Can you work these out from the model? Positions are in its coordinate system, mm. A direction names the side the tool comes from. Coordinates: 2 decimals unless noted, no trailing zeros. Order: outer loops, then holes, each group sorted by start corner. A loop starts at its lowest first (then second) coordinate and runs counter-clockwise, first axis right, second up. Notation, with made-up numbers: (50.25, 35.5) -> (87.25, 35.5) arc R12 ccw to (87.25, 47.5) -> close; hole circle Ø3 at (38, 14). An arc over 180 degrees is marked (long way). Answer in a Markdown table with one row per item. Add a question column.
1. Will these pins go through, and if not, where does the flat tip stop? pin 1 (2 mm diameter, centred on x = -3.5, y = 0.5, fed in from -Z); pin 2 (1.5 mm diameter, centred on x = 5.5, z = -7, fed in from -Y).
2. On a 3-axis mill with a long thin cutter (end or side, diameter ignored), from which of +Z, -Z, +X, -X, +Y, -Y can I reach the whole of each face in a straight line? I mean faces 4 (the face through (-6.987, -2.2, -7.466)), 5 (the face through (6.465, -6.39, -6.42)). Say none if no direction works.
3. If I drill on line 1 along X through (y, z) = (0, -3.5); line 2 along Z through (x, y) = (7.25, 2.25), over which ranges is the centre line in solid material (lowest first)? Write a range as [from, to].
4. Imagine slicing it at C-C on z = -6. Write out the boundary of the cut face in (x, y), plus the area to 3 significant figures.
5. We'd pull the mould along X, two halves only. Please class faces 1 (the face through (0, -9.146, -3)), 2 (the face through (0, 5, -4)), 3 (the face through (6.505, -6.43, -3.197)): pulls with the +X half, pulls with the -X half, needs draft (parallel to the pull), parting line crosses it, or undercut.
Autodesk Inventor part; units mm, degrees
ref_plane "YZ Plane" through (0, 0, 0) normal (1, 0, 0) x (0, 1, 0)
ref_plane "XZ Plane" through (0, 0, 0) normal (0, 1, 0) x (-1, 0, 0)
ref_plane "XY Plane" through (0, 0, 0) normal (0, 0, 1) x (1, 0, 0)
sketch "Sketch1" plane through (0, 0, 0) normal (0, 0, 1) x (1, 0, 0)
  line L0 (-12.8051, 0) -> (12.8051, 0)
  line L1 (9.1465, -3.7886) -> (3.7886, -9.1465)
  line L2 (3.7886, -9.1465) -> (-3.7886, -9.1465)
  line L3 (-3.7886, -9.1465) -> (-9.1465, -3.7886)
  line L4 (-9.1465, -3.7886) -> (-9.1465, 3.7886)
  line L5 (-9.1465, 3.7886) -> (-3.7886, 9.1465)
  line L6 (-3.7886, 9.1465) -> (3.7886, 9.1465)
  line L7 (3.7886, 9.1465) -> (9.1465, 3.7886)
  line L8 (9.1465, 3.7886) -> (9.1465, -3.7886)
  circle A0 centre (0, 0) radius 5
  point P0 (9.1465, 0)
  dimension "d0" = 18.293
  dimension "d1" = 10
extrude "Extrusion1" add sketch "Sketch1" against normal blind 6.48 contours L4 L5 L6 L7 L8 L0 A0 | L0 A0 L8 L1 L2 L3 L4
sketch "Sketch2" plane through (0, 0, -6.48) normal (0, 0, -1) x (-1, 0, 0)
  circle A0 centre (0, 0) radius 5
  circle A1 centre (0, 0) radius 7.325
  dimension "d4" = 14.65
extrude "Extrusion2" add sketch "Sketch2" along normal blind 2
fillet "Fillet1" radius 0.2 17 edges at (0, -9.1465, 0) (-6.4676, -6.4676, 0) (6.4676, -6.4676, 0) (9.1465, 0, 0) (6.4676, 6.4676, 0) (0, 9.1465, 0) (-6.4676, 6.4676, 0) (-9.1465, 0, 0) (9.1465, 0, -6.48) (6.4676, -6.4676, -6.48) (0, -9.1465, -6.48) (-6.4676, -6.4676, -6.48) (-9.1465, 0, -6.48) (-6.4676, 6.4676, -6.48) (0, 9.1465, -6.48) (6.4676, 6.4676, -6.48) (-5, 0, 0)
thread "Thread1"
properties part number "201-11" material "Steel"
Answers follow:
| question | item | result |
|---|---|---|
| 1 | pin 1 | passes through |
| 1 | pin 2 | stops at y = -7.83 |
| 2 | face 4 | -Z |
| 2 | face 5 | -Z, +X, -Y |
| 3 | line 1 | x = [-9.15, -5], [5, 9.15] |
| 3 | line 2 | z = [-6.48, 0] |
| 4 | outline | (-9.15, -3.79) -> (-3.79, -9.15) -> (3.79, -9.15) -> (9.15, -3.79) -> (9.15, 3.79) -> (3.79, 9.15) -> (-3.79, 9.15) -> (-9.15, 3.79) -> close; hole circle Ø10 at (0, 0) |
| 4 | area | 199 mm² |
| 5 | face 1 | needs draft |
| 5 | face 2 | undercut |
| 5 | face 3 | pulls with the +X half |
